```python
from build123d import *

# Parameters (mm, degrees)
BOSS_EXTRUDE1_DEPTH = 38.1
FILLET1_R           = 0.5


with BuildPart() as part:
    # Sketch1 → Boss-Extrude1 (new, symmetric)
    with BuildSketch(Plane.XY):
        Polygon((7.332348419, 0), (3.666174209, 6.35), (-3.666174209, 6.35), (-7.332348419, 0), (-3.666174209, -6.35), (3.666174209, -6.35), align=None)
    extrude(amount=BOSS_EXTRUDE1_DEPTH, both=True)

    # Fillet1
    fillet1_edges = [part.edges().sort_by_distance(p)[0] for p in [
        (3.666174209, -6.35, 0),
        (-3.666174209, -6.35, 0),
        (-7.332348419, 0, 0),
        (-3.666174209, 6.35, 0),
        (3.666174209, 6.35, 0),
        (7.332348419, 0, 0),
    ]]
    fillet(fillet1_edges, radius=FILLET1_R)


solid = part.part
```
Read the model definition and answer for the solid it produces. Units are mm, in the model's axes. Coordinates: 2 decimals unless noted, no trailing zeros. Loops run counter-clockwise (first coordinate to the right, second up) from the corner with the lowest first, then second, coordinate; pieces in that order, holes last. Notation, with made-up numbers: (53.25, 87) -> (101.25, 87) arc R15 ccw to (101.25, 112) -> close; hole circle Ø2 at (77.25, 37.5). An arc over 180 degrees is marked (long way). Return JSON: item names as keys, results as strings.
Item 1: Find the intervals of material crossed by probe 1 along Y at (x, z) = (-4, -9); probe 2 along Y at (x, z) = (5, 29); probe 3 along X at (y, z) = (-5, 26.5), in increasing order.
Answers:
{"probe 1": "y = -5.77 to 5.77", "probe 2": "y = -4.04 to 4.04", "probe 3": "x = -4.45 to 4.45"}
Item 2: A flat-ended cylindrical pin translates along its axis: P1, Ø3, axis at y = 3, z = -18, coming from the +X side. Find the tip coordinate at first contact, or state that the pin passes through.
Answers:
{"P1": "stops at x = 6.47"}
Item 3: Find section B-B (y = -1). Determine the outline of the cut face in (x, z) (3 decimals).
Answers:
{"outline": "(-6.755, -38.1) -> (6.755, -38.1) -> (6.755, 38.1) -> (-6.755, 38.1) -> close"}
Item 4: Find section C-C (x = -6). Determine the outline of the cut face in (y, z).
Answers:
{"outline": "(-2.31, -38.1) -> (2.31, -38.1) -> (2.31, 38.1) -> (-2.31, 38.1) -> close"}
